from build123d import *

# Parameters (mm, degrees)
F0_W     = 101.6
F0_H     = 71.12
F1_DEPTH = 101.6
F2_W     = 81.28
F2_H     = 71.12
F3_DEPTH = 81.28
F4_W     = 33.02
F4_H     = 45.72
F5_DEPTH = 20.321
F6_W     = 33.02
F6_H     = 45.72
F7_DEPTH = 20.321


with BuildPart() as f1:
    # F0 (on Front) → F1 (new body)
    with BuildSketch(Plane.XZ):
        Rectangle(F0_W, F0_H)
    extrude(amount=F1_DEPTH)

    # F2 (on face) → F3 (cut)
    with BuildSketch(Plane.XZ.offset(101.6)):
        with Locations((10.16, 0)):
            Rectangle(F2_W, F2_H)
    extrude(amount=-F3_DEPTH, mode=Mode.SUBTRACT)

    # F4 (on face) → F5 (cut, through all)
    with BuildSketch(Plane.XZ.offset(20.32)):
        with Locations((10.16, 0)):
            Rectangle(F4_W, F4_H)
    extrude(amount=-F5_DEPTH, mode=Mode.SUBTRACT)

    # F6 (on face) → F7 (cut, through all)
    with BuildSketch(Plane.YZ.offset(-30.48)):
        with Locations((-60.96, 0)):
            Rectangle(F6_W, F6_H)
    extrude(amount=-F7_DEPTH, mode=Mode.SUBTRACT)


solid = f1.part
Geometry: final body of the model. Coordinates: model frame, mm. A direction names the side the tool comes from. Give positions to 0.01 mm unless a question says otherwise; leave off trailing zeros. Order: outer loops, then holes, each group sorted by start corner. A loop starts at its lowest first (then second) coordinate and runs counter-clockwise, first axis right, second up. Notation, with made-up numbers: (89.25, 18.25) -> (112.25, 18.25) arc R17 cw to (112.25, 29.25) -> close; hole circle Ø5 at (-29.5, 44.25). An arc over 180 degrees is marked (long way). Put each result on its own line as item: value.
Q1. Draft query along Y for faces 1 (the face through (-12, 0, 0)), 2 (the face through (10, -10, -22.86)), 3 (the face through (-40, -61, 22.86)). Return one class per face: released by +Y, released by -Y, zero draft, split by the parting line, or undercut.
Here are the results:
face 1: released by +Y
face 2: zero draft
face 3: undercut
Q2. Section A-A, the plane y = -56.5. Return loops of the section in (x, z), then the cut area to 3 significant figures.
Here are the results:
outline: (-50.8, -35.56) -> (-30.48, -35.56) -> (-30.48, -22.86) -> (-50.8, -22.86) -> close; (-50.8, 22.86) -> (-30.48, 22.86) -> (-30.48, 35.56) -> (-50.8, 35.56) -> close
area: 516 mm^2
Q3. Reachability of faces 4 (the face through (-40, -44.45, 0)), 5 (the face through (-6.35, -10, 0)), 6 (the face through (-8, -20.32, 0)) from +Z, -Z, +X, -X, +Y, -Y: full face, straight path, thin tool, end or side. Return the list, or none.
Here are the results:
face 4: +X, -X
face 5: +Y, -Y
face 6: +Z, -Z, +X, -Y
Q4. Pin query (flat end, axial travel): pin 1 (22.5 mm diameter, centred on x = -45, z = -3.5, fed in from +Y); pin 2 (6 mm diameter, centred on y = -45.5, z = 15.5, fed in from +X); pin 3 (4 mm diameter, centred on x = 24, z = 6.5, fed in from -Y); pin 4 (6 mm diameter, centred on x = 34.5, z = -13, fed in from -Y). Return the tip coordinate at first contact, or that it passes through.
Here are the results:
pin 1: stops at y = 0
pin 2: stops at x = -30.48
pin 3: passes through
pin 4: stops at y = -20.32
Q5. Material intervals for L1, parallel to X at y = -39.5, z = -5; L2, parallel to Y at x = 31.5, z = -21; L3, parallel to Z at x = -45.5, y = -54.5, sorted ascending.
Here are the results:
L1: x = -50.8 to -30.48
L2: y = -20.32 to 0
L3: z = -35.56 to -22.86, 22.86 to 35.56
Q6. Section C-C, the plane z = -14. Return loops of the section in (x, y), then the cut area to 3 significant figures.
Here are the results:
outline: (-50.8, -101.6) -> (-30.48, -101.6) -> (-30.48, -77.47) -> (-50.8, -77.47) -> close; (-50.8, -44.45) -> (-30.48, -44.45) -> (-30.48, -20.32) -> (-6.35, -20.32) -> (-6.35, 0) -> (-50.8, 0) -> close; (26.67, -20.32) -> (50.8, -20.32) -> (50.8, 0) -> (26.67, 0) -> close
area: 2,370 mm^2
Q7. Section B-B, the plane x = -4.5. Return loops of the section in (y, z).
Here are the results:
outline: (-20.32, -35.56) -> (0, -35.56) -> (0, -22.86) -> (-20.32, -22.86) -> close; (-20.32, 22.86) -> (0, 22.86) -> (0, 35.56) -> (-20.32, 35.56) -> close
Q8. Section D-D, the plane y = -8.5. Return loops of the section in (x, z), then the cut area to 3 significant figures.
Here are the results:
outline: (-50.8, -35.56) -> (50.8, -35.56) -> (50.8, 35.56) -> (-50.8, 35.56) -> close; hole (-6.35, -22.86) -> (26.67, -22.86) -> (26.67, 22.86) -> (-6.35, 22.86) -> close
area: 5,720 mm^2
